Input: part model. Units: mm. Frame: model coordinates. A direction names the side the tool comes from. Coordinates: 2 decimals unless noted, no trailing zeros. Order: outer loops, then holes, each group sorted by start corner. A loop starts at its lowest first (then second) coordinate and runs counter-clockwise, first axis right, second up. Notation, with made-up numbers: M -37,71 L 20,71 A25 cw 20,100 Z; hole C 71,75.5 d4. An arc over 180 degrees is marked long. One line per item, written item: value.
```python
from build123d import *

# Parameters (mm, degrees)
BOSS_EXTRUDE1_DEPTH = 10
SKETCH2_R           = 2
SKETCH2_R_2         = 1
BOSS_EXTRUDE2_DEPTH = 3


with BuildPart() as part:
    # Sketch1 → Boss-Extrude1 (new body)
    with BuildSketch(Plane(origin=(0, 0, 0), x_dir=(1, 0, 0), z_dir=(0, 1, 0))):
        with BuildLine():
            Line((-4.171572875, -7), (4.171572875, -7))
            ThreePointArc((4.171572875, -7), (7, -7), (7, -4.171572875))
            Line((7, -4.171572875), (7, 4.171572875))
            ThreePointArc((7, 4.171572875), (7, 7), (4.171572875, 7))
            Line((4.171572875, 7), (-4.171572875, 7))
            ThreePointArc((-4.171572875, 7), (-7, 7), (-7, 4.171572875))
            Line((-7, 4.171572875), (-7, -4.171572875))
            ThreePointArc((-7, -4.171572875), (-7, -7), (-4.171572875, -7))
        make_face()
    extrude(amount=BOSS_EXTRUDE1_DEPTH)

    # Sketch2 → Boss-Extrude2 (add)
    with BuildSketch(Plane.XZ):
        with Locations(Location((0, 0, 0), (0, 0, 90))):
            Circle(SKETCH2_R)
        with Locations(Location((-5.08, 0, 0), (0, 0, 90))):
            Circle(SKETCH2_R_2)
        with Locations(Location((5.08, 0, 0), (0, 0, 90))):
            Circle(SKETCH2_R_2)
    extrude(amount=BOSS_EXTRUDE2_DEPTH)


solid = part.part
```
(1) Ray query, line 1 (X direction, y = -0.5, z = -0.5); line 2 (X direction, y = 4, z = -3.5); line 3 (Y direction, x = -1.25, z = 3). Return the intervals inside material, ascending. Write a range as from..to.
Data:
line 1: x = -5.95..-4.21, -1.94..1.94, 4.21..5.95
line 2: x = -7..7
line 3: y = 0..10
(2) Cut plane B-B on y = -1.75. Output: boundary loops of the cut face in (x, z).
Data:
outline: C -5.08,0 d2; C 0,0 d4; C 5.08,0 d2
(3) Draft query along Z for faces 1 (the flat face through (0, 5, 7)), 2 (the cylindrical face through (2, -1, 0)), 3 (the cylindrical face through (-7, 5, 7)). Return one class per face: released by +Z, released by -Z, zero draft, split by the parting line, or undercut.
Data:
face 1: released by +Z
face 2: split by the parting line
face 3: undercut
(4) Access query for faces 4 (the flat face through (2, 0, -2)), 5 (the flat face through (0, -3, 0)), 6 (the flat face through (-7, 5, 0)), 7 (the flat face through (0, 5, -7)), 8 (the flat face through (7, 5, 0)). Directions: +Z, -Z, +X, -X, +Y, -Y. A direction counts if a zero-diameter tool reaches every point of the face in a straight line with its end or side. Return the directions, or none.
Data:
face 4: -Y
face 5: +Z, -Z, +X, -X, -Y
face 6: -X, +Y, -Y
face 7: -Z, +Y, -Y
face 8: +X, +Y, -Y
(5) Cut plane C-C on y = 5. Output: boundary loops of the cut face in (x, z), plus the area to 3 significant figures.
Data:
outline: M -7,-4.17 A2 ccw -4.17,-7 L 4.17,-7 A2 ccw 7,-4.17 L 7,4.17 A2 ccw 4.17,7 L -4.17,7 A2 ccw -7,4.17 Z
area: 205 mm2
(6) First-contact query: pin 1 (1 mm diameter, centred on y = 1.5, z = 4, fed in from +X); pin 2 (4 mm diameter, centred on x = 3.5, z = -3.5, fed in from -Y); pin 3 (6.5 mm diameter, centred on x = -1.5, y = 7, fed in from -Z). Flat tips, straight axial feed; report the tip coordinate or a pass-through.
Data:
pin 1: stops at x = 7.27
pin 2: stops at y = 0
pin 3: stops at z = -7.4
(7) Cut plane A-A on z = 0. Output: boundary loops of the cut face in (x, y), plus the area to 3 significant figures.
Data:
outline: M -7,0 L -6.08,0 L -6.08,-3 L -4.08,-3 L -4.08,0 L -2,0 L -2,-3 L 2,-3 L 2,0 L 4.08,0 L 4.08,-3 L 6.08,-3 L 6.08,0 L 7,0 L 7,10 L -7,10 Z
area: 164 mm2
(8) Cut plane D-D on x = 0. Output: boundary loops of the cut face in (y, z).
Data:
outline: M -3,-2 L 0,-2 L 0,-7 L 10,-7 L 10,7 L 0,7 L 0,2 L -3,2 Z
